from build123d import *

# Parameters (mm, degrees)
F0_W     = 50.8
F0_H     = 31.75
F1_DEPTH = 31.75
F2_W     = 19.05
F2_H     = 19.05
F3_DEPTH = 19.05
F4_W     = 19.05
F4_H     = 19.05
F5_DEPTH = 31.751
F6_W     = 19.05
F6_H     = 12.7
F7_DEPTH = 31.75
F9_DEPTH = 50.871556


with BuildPart() as f1:
    # F0 (on Front) → F1 (new body)
    with BuildSketch(Plane.XZ):
        with Locations((25.4, 15.875)):
            Rectangle(F0_W, F0_H)
    extrude(amount=-F1_DEPTH)

    # F2 (on Right) → F3 (cut)
    with BuildSketch(Plane.YZ):
        with Locations((22.394827, 22.882153)):
            Rectangle(F2_W, F2_H)
    extrude(amount=F3_DEPTH, mode=Mode.SUBTRACT)

    # F4 (on Top) → F5 (cut, through all)
    with BuildSketch(Plane.XY):
        with Locations((41.275, 22.261919)):
            Rectangle(F4_W, F4_H)
    extrude(amount=F5_DEPTH, mode=Mode.SUBTRACT)

    # F6 (on Front) → F7 (join)
    with BuildSketch(Plane.XZ):
        with Locations((41.345556, 6.35)):
            Rectangle(F6_W, F6_H)
    extrude(amount=-F7_DEPTH)

    # F8 (on Right) → F9 (cut, through all)
    with BuildSketch(Plane.YZ):
        Polygon((31.830321, 32.020881), (12.781355, 31.822454), (31.830321, 12.970881), align=None)
    extrude(amount=F9_DEPTH, mode=Mode.SUBTRACT)


solid = f1.part
Verification items for the finished model (mm, model axes). A direction names the side the tool comes from. Give positions to 0.01 mm unless a question says otherwise; leave off trailing zeros. Loops run counter-clockwise (first coordinate to the right, second up) from the corner with the lowest first, then second, coordinate; pieces in that order, holes last.
1) Set-up check for faces 1 (the flat face through (9, 12.87, 22)), 2 (the flat face through (25, 16, 0)), 3 (the flat face through (50.8, 6, 22)): record each of +Z, -Z, +X, -X, +Y, -Y from which the full face is reachable in a straight line by a thin tool's end or side.
2) Depth check by flat-ended pin: pin 1 Ø4 at (x, y) = (8, 26.5) entering from +Z; pin 2 Ø10 at (x, z) = (10.5, 23.5) entering from +Y; pin 3 Ø5.5 at (y, z) = (21, 22) entering from -X. Enter the tip coordinate at first touch or a pass-through.
3) Sectioned sample at B-B, the plane z = 16.5. Enter the section's corners in (x, y), then the cut area to 3 significant figures.
4) Sectioned sample at D-D, the plane y = 26. Enter the section's corners in (x, z), then the cut area to 3 significant figures.
5) Sectioned sample at A-A, the plane y = 22.5. Enter the section's corners in (x, z), then the cut area to 3 significant figures.
6) Thickness scan on line 1 along X through (y, z) = (11.5, 29.5); line 2 along Y through (x, z) = (11, 20); line 3 along Y through (x, z) = (39.5, 22). Record the ranges inside material, lowest first.
Answers:
1. face 1: +Z, -X, +Y
1. face 2: -Z, +X, -X, +Y, -Y
1. face 3: +Z, +X, +Y, -Y
2. pin 1: stops at z = 13.36
2. pin 2: stops at y = 12.87
2. pin 3: stops at x = 19.05
3. outline: (0, 0) - (50.8, 0) - (50.8, 12.74) - (31.75, 12.74) - (31.75, 28.26) - (19.05, 28.26) - (19.05, 12.87) - (0, 12.87) - close
3. area: 847 mm2
4. outline: (0, 0) - (31.75, 0) - (31.75, 18.74) - (19.05, 18.74) - (19.05, 13.36) - (0, 13.36) - close; (31.82, 0) - (50.87, 0) - (50.87, 12.7) - (31.82, 12.7) - close
4. area: 734 mm2
5. outline: (0, 0) - (31.75, 0) - (31.75, 22.2) - (19.05, 22.2) - (19.05, 13.36) - (0, 13.36) - close; (31.82, 0) - (50.87, 0) - (50.87, 12.7) - (31.82, 12.7) - close
5. area: 778 mm2
6. line 1: x = 0 to 50.8
6. line 2: y = 0 to 12.87
6. line 3: y = 0 to 12.74
